from build123d import *

# Parameters (mm, degrees)
SKETCH006_W     = 55.805504
SKETCH006_H     = 42.953331
SKETCH006_W_2   = 24
SKETCH006_H_2   = 23
PAD003_DEPTH    = 3
CHAMFER001_SIZE = 1
CHAMFER002_SIZE = 2.4


with BuildPart() as part:
    # Sketch006 → Pad003 (new body)
    with BuildSketch(Plane.XY):
        with Locations((1.3612, 4.995676)):
            Rectangle(SKETCH006_W, SKETCH006_H)
        with Locations((1.122957, 3.1348)):
            Rectangle(SKETCH006_W_2, SKETCH006_H_2, mode=Mode.SUBTRACT)
    extrude(amount=PAD003_DEPTH)

    # Chamfer001
    chamfer001_edges = [part.edges().sort_by_distance(p)[0] for p in [
        (1.3612, -16.480989, 3),
        (29.263952, 4.995676, 3),
        (1.3612, 26.472342, 3),
        (-26.541552, 4.995677, 3),
        (1.3612, -16.480989, 0),
        (29.263952, 4.995676, 0),
        (1.3612, 26.472342, 0),
        (-26.541552, 4.995677, 0),
    ]]
    chamfer(chamfer001_edges, length=CHAMFER001_SIZE)

    # Chamfer002
    chamfer002_edges = [part.edges().sort_by_distance(p)[0] for p in [
        (1.122957, 14.6348, 3),
        (13.122957, 3.1348, 3),
        (1.122957, -8.3652, 3),
        (-10.877043, 3.1348, 3),
    ]]
    chamfer(chamfer002_edges, length=CHAMFER002_SIZE)


solid = part.part
For this review, take the finished solid that the model builds, in its own axes (mm). A direction names the side the tool comes from. Round coordinates to 2 decimals unless told otherwise and drop trailing zeros. Loops run counter-clockwise (first coordinate to the right, second up) from the corner with the lowest first, then second, coordinate; pieces in that order, holes last. Notation, with made-up numbers: (57, -6.75) - (73, -6.75) arc R21 ccw to (73, 24.25) - close; hole circle Ø8 at (72.25, 58.25). An arc over 180 degrees is marked (long way). Put each result on its own line as item: value. Start each with the question number.
1. For probe 1 along X at (y, z) = (3, 2.7); probe 2 along X at (y, z) = (11.5, 2.75); probe 3 along Y at (x, z) = (-1, 2.1), list the stretches that pass through material, from the lowest coordinate up. Write a range as [from, to].
2. Consider section C-C on z = 2.5. State the section outline as (x, y) points.
3. For faces 3 (the flat face through (-12.06, 2.94, 1.783)), 4 (the flat face through (1, 19, 0)), list the 3-axis set-ups (+Z, -Z, +X, -X, +Y, -Y) from which the entire face can be reached by the end or side of a thin tool; tool diameter is ignored.
4. Mouldability with a two-part tool opening along X and no side actions: class faces 1 (the flat face through (0.921, 15.818, 1.783)), 2 (the flat face through (1, 19, 3)) as +X half, -X half, draft (parallel to the pull), parting line (faces both ways), or undercut.
5. Insertion check: P1, Ø0.7, axis at y = 4.5, z = 0, coming from the +X side; P2, Ø0.7, axis at x = -5, z = 0.5, coming from the +Y side. Each pin has a flat end and moves straight along its axis. Give the tip position at first contact, or say it passes through.
6. Consider section D-D on x = 20. State the section outline as (y, z) points, plus the area to 3 significant figures.
7. Consider section B-B on y = -5. State the section outline as (x, z) points.
8. Consider section A-A on x = -1.5. State the section outline as (y, z) points.
Result sheet:
1. probe 1: [-25.84, -12.98], [15.22, 28.56]
1. probe 2: [-25.79, -13.03], [15.27, 28.51]
1. probe 3: [-16.38, -9.87], [16.13, 26.37]
2. outline: (-26.04, -15.98) - (28.76, -15.98) - (28.76, 25.97) - (-26.04, 25.97) - close; hole (-12.78, -10.27) - (15.02, -10.27) - (15.02, 16.53) - (-12.78, 16.53) - close
3. face 3: +Z
3. face 4: -Z, +X, -X, +Y, -Y
4. face 1: undercut
4. face 2: draft
5. P1: x = 28.61
5. P2: y = 26.32
6. outline: (-16.48, 1) - (-15.48, 0) - (25.47, 0) - (26.47, 1) - (26.47, 2) - (25.47, 3) - (-15.48, 3) - (-16.48, 2) - close
6. area: 127 mm^2
7. outline: (-26.54, 1) - (-25.54, 0) - (-10.88, 0) - (-10.88, 0.6) - (-13.28, 3) - (-25.54, 3) - (-26.54, 2) - close; (13.12, 0) - (28.26, 0) - (29.26, 1) - (29.26, 2) - (28.26, 3) - (15.52, 3) - (13.12, 0.6) - close
8. outline: (-16.48, 1) - (-15.48, 0) - (-8.37, 0) - (-8.37, 0.6) - (-10.77, 3) - (-15.48, 3) - (-16.48, 2) - close; (14.63, 0) - (25.47, 0) - (26.47, 1) - (26.47, 2) - (25.47, 3) - (17.03, 3) - (14.63, 0.6) - close
